Geometry check sheet. Reference: the model listing, model coordinates, mm. A direction names the side the tool comes from. Give positions to 0.01 mm unless a question says otherwise; leave off trailing zeros. Write each loop counter-clockwise with the first axis right and the second up, starting at its lowest first coordinate (ties: lowest second). Pieces come first, ordered by that corner, then holes.
(1) Thickness scan on line 1 along Z through (x, y) = (95.75, 19.6); line 2 along X through (y, z) = (15, 0); line 3 along X through (y, z) = (19.7, -13.75). Record the ranges inside material, lowest first.
(2) Cross-section at D-D (y = 12). Record the boundary of the cut face in (x, z).
(3) Cross-section at C-C (z = 0). Record the boundary of the cut face in (x, y), and give its area (4 significant figures).
(4) Mould release check, pull along Z, two halves, no side actions. Record for faces 5 (the flat face through (0, 4, 65.5)), 6 (the flat face through (2.5, 3, 68)), 7 (the flat face through (58, 16, 4.5)): +Z half, -Z half, draft (parallel to the pull), parting line (faces both ways), or undercut.
(5) Cross-section at A-A (x = 95.75). Record the boundary of the cut face in (y, z).
(6) Depth check by flat-ended pin: P1, Ø5, axis at y = 2.5, z = -67.5, coming from the +X side; P2, Ø1.5, axis at y = 3.5, z = 24, coming from the +X side; P3, Ø8, axis at x = -31, y = 6.5, coming from the -Z side; P4, Ø14, axis at x = 95.75, z = -13.75, coming from the -Y side. Enter the tip coordinate at first touch or a pass-through.
(7) Cross-section at B-B (x = 0). Record the boundary of the cut face in (y, z).
(8) Tool access check on faces 1 (the flat face through (-3, 20, 57)), 2 (the flat face through (0, 7, -68)), 3 (the flat face through (-2.5, 4, 68)), 4 (the flat face through (84, 19, 0)). Record the directions out of +Z, -Z, +X, -X, +Y, -Y that give a thin tool (end or side, any length) a straight path to the whole face; none if there is none.
Autodesk Inventor part; units mm, degrees
ref_plane "Pracovní rovina2" through (0, 0, 54.5) normal (0, 0, 1) x (1, 0, 0)
ref_plane "Pracovní rovina3" through (0, 0, -54.5) normal (0, 0, 1) x (1, 0, 0)
ref_plane "Pracovní rovina4" through (54.5, 0, 0) normal (1, 0, 0) x (0, 1, 0)
sketch "Náčrt1" plane through (0, 0, 0) normal (0, 1, 0) x (-1, 0, 0)
  circle A0 centre (0, 0) radius 55
  line L0 (0, -70) -> (26.9258, -70)
  line L1 (0, -70) -> (-26.9258, -70)
  line L2 (-70, 0) -> (-70, -26.9258)
  line L3 (-70, 0) -> (-70, 26.9258)
  line L4 (70, 0) -> (70, -26.9258)
  line L5 (70, 0) -> (70, 26.9258)
  line L6 (0, 70) -> (26.9258, 70)
  line L7 (0, 70) -> (-26.9258, 70)
  line L8 (-104.3981, 0) -> (104.3981, 0)
  line L9 (0, -104.3981) -> (0, 104.3981)
  arc A1 (26.9258, -70) -> (70, -26.9258) centre (0, 0) ccw
  arc A2 (-70, -26.9258) -> (-26.9258, -70) centre (0, 0) ccw
  arc A3 (70, 26.9258) -> (26.9258, 70) centre (0, 0) ccw
  arc A4 (-26.9258, 70) -> (-70, 26.9258) centre (0, 0) ccw
  dimension "d1" = 110
extrude "Vysunutí1" add sketch "Náčrt1" along normal blind 25 contours L8 L4 A1 L0 L9 A0 | A0 L9 L6 A3 L5 L8 | A0 L8 L3 A4 L7 L9 | L9 L1 A2 L2 L8 A0
sketch "Náčrt2" plane through (-26.9258, 0, 70) normal (0, 0, 1) x (1, 0, 0)
  line L0 (53.8516, 0) -> (0, 0)
  line L1 (24.4258, 0) -> (29.4258, 0)
  line L2 (29.4258, 0) -> (29.4258, 7)
  line L3 (29.4258, 7) -> (24.4258, 7)
  line L4 (24.4258, 7) -> (24.4258, 0)
  line L5 (96.9258, 0) -> (96.9258, 25)
  point P0 (26.9258, 0)
  dimension "d5" = 5
  dimension "d6" = 7
  dimension "d7" = 67.5
extrude "Vysunutí2" cut sketch "Náčrt2" against normal blind 4.5
sketch "Náčrt3" plane through (26.9258, 0, -70) normal (0, 0, -1) x (-1, 0, 0)
  line L0 (0, 0) -> (53.8516, 0)
  line L1 (53.8516, 0) -> (53.8516, 25)
  line L2 (0, 25) -> (53.8516, 25)
  line L3 (0, 0) -> (0, 25)
  line L4 (53.8516, 0) -> (96.9258, 0)
  line L5 (96.9258, 0) -> (96.9258, 25)
  line L6 (53.8516, 25) -> (96.9258, 25)
  line L7 (53.8516, 0) -> (53.8516, 25)
  line L8 (24.4258, 0) -> (0, 0)
  line L9 (24.4258, 0) -> (29.4258, 0)
  line L10 (29.4258, 0) -> (29.4258, 7)
  line L11 (29.4258, 7) -> (24.4258, 7)
  line L12 (24.4258, 7) -> (24.4258, 0)
  point P0 (26.9258, 0)
  dimension "d10" = 5
  dimension "d11" = 7
  dimension "d12" = 67.5
extrude "Vysunutí3" cut sketch "Náčrt3" against normal blind 4.5 contours L12 L11 L10 L0
sketch "Náčrt4" plane through (0, 25, 0) normal (0, 1, 0) x (1, 0, 0)
  line L0 (70, -26.9258) -> (70, 26.9258)
  line L1 (70, -4.5) -> (52.6737, -4.5)
  line L2 (52.6737, -4.5) -> (52.6737, 4.5)
  line L3 (52.6737, 4.5) -> (70, 4.5)
  line L4 (70, 4.5) -> (70, -4.5)
  line L5 (-98, 0) -> (98, 0)
  line L6 (0, 98) -> (0, -98)
  point P0 (0, 0)
  point P1 (70, 4.5)
  dimension "d15" = 9
  dimension "d16" = 4.5
extrude "Vysunutí4" cut sketch "Náčrt4" against normal blind 4
ref_plane "Pracovní rovina2" through (0, 0, 54.5) normal (0, 0, 1) x (1, 0, 0)
sketch "Náčrt6" plane through (0, 0, 54.5) normal (0, 0, 1) x (1, 0, 0)
  line L0 (-26.9258, 25) -> (26.9258, 25)
  line L1 (3, 25) -> (-3, 25)
  line L2 (-3, 25) -> (-3, 15)
  line L3 (-3, 15) -> (3, 15)
  line L4 (3, 15) -> (3, 25)
  line L5 (0, 30) -> (0, -5)
  point P0 (0, 0)
  dimension "d21" = 6
  dimension "d22" = 10
extrude "Vysunutí5" cut sketch "Náčrt6" along normal blind 4.5
ref_plane "Pracovní rovina3" through (0, 0, -54.5) normal (0, 0, 1) x (1, 0, 0)
sketch "Náčrt7" plane through (0, 0, -54.5) normal (0, 0, 1) x (1, 0, 0)
  line L0 (-55, 25) -> (54.8156, 25)
  line L1 (2.5, 25) -> (-2.5, 25)
  line L2 (-2.5, 25) -> (-2.5, 15)
  line L3 (-2.5, 15) -> (2.5, 15)
  line L4 (2.5, 15) -> (2.5, 25)
  line L5 (0, 30) -> (0, -5)
  point P0 (0, 0)
  point P1 (-3, 25)
  dimension "d26" = 5
  dimension "d27" = 10
extrude "Vysunutí6" cut sketch "Náčrt7" against normal blind 4.5
sketch "Náčrt8" plane through (70, 0, 26.9258) normal (1, 0, 0) x (0, 0, -1)
  line L0 (3.4258, 21) -> (50.4258, 21)
  line L1 (50.4258, 21) -> (50.4258, 19)
  line L2 (50.4258, 19) -> (3.4258, 19)
  line L3 (3.4258, 19) -> (3.4258, 21)
  line L4 (31.4258, 21) -> (22.4258, 21)
  line L5 (53.8516, 25) -> (0, 25)
  line L6 (26.9258, 25) -> (26.9258, 9.9917)
  point P0 (26.9258, 0)
  dimension "d30" = 47
  dimension "d31" = 2
extrude "Vysunutí7" add sketch "Náčrt8" along normal blind 37
sketch "Náčrt9" plane through (0, 21, 0) normal (0, 1, 0) x (1, 0, 0)
  circle A0 centre (95.75, -13.75) radius 8.75
  circle A1 centre (95.75, 13.75) radius 8.75
  line L0 (-105.4, 0) -> (142.4, 0)
  line L1 (107, 23.5) -> (107, -23.5)
  point P0 (0, 0)
  dimension "d34" = 17.5
  dimension "d35" = 17.5
  dimension "d37" = 5
  dimension "d38" = 5
  dimension "d41" = 11.25
  dimension "d42" = 11.25
extrude "Vysunutí8" cut sketch "Náčrt9" against normal blind 27
ref_plane "Pracovní rovina4" through (54.5, 0, 0) normal (1, 0, 0) x (0, 1, 0)
sketch "Náčrt10" plane through (54.5, 0, 0) normal (1, 0, 0) x (0, 1, 0)
  line L0 (0, 55) -> (0, -55)
  line L1 (21, -4.5) -> (0, -4.5)
  line L2 (0, -4.5) -> (0, 4.5)
  line L3 (0, 4.5) -> (21, 4.5)
  line L4 (21, 4.5) -> (21, -4.5)
  point P0 (0, 0)
  dimension "d44" = 9
extrude "Vysunutí9" cut sketch "Náčrt10" along normal blind 4
properties part number "Kruh"
Reply:
1. line 1: z = -23.5 to -22.5, -5 to 5, 22.5 to 23.5
1. line 2: x = -70 to -55, 58.5 to 70
1. line 3: x = -70 to -53.25, 53.25 to 87, 104.5 to 107
2. outline: (-70, -26.93) arc R75 ccw to (-26.93, -70) - (26.93, -70) arc R75 ccw to (70, -26.93) - (70, 26.93) arc R75 ccw to (26.93, 70) - (-26.93, 70) arc R75 ccw to (-70, 26.93) - close; hole (54.82, -4.5) - (58.5, -4.5) - (58.5, 4.5) - (54.82, 4.5) arc R55 ccw (long way) to start
3. outline: (-70, 0) - (-55, 0) - (-55, 25) - (-70, 25) - close; (58.5, 0) - (70, 0) - (70, 19) - (107, 19) - (107, 21) - (58.5, 21) - close
3. area: 690.5 mm2
4. face 5: +Z half
4. face 6: draft
4. face 7: undercut
5. outline: (19, -23.5) - (21, -23.5) - (21, -22.5) - (19, -22.5) - close; (19, -5) - (21, -5) - (21, 5) - (19, 5) - close; (19, 22.5) - (21, 22.5) - (21, 23.5) - (19, 23.5) - close
6. P1: stops at x = 37.42
6. P2: stops at x = 70
6. P3: stops at z = -69.97
6. P4: passes through
7. outline: (0, -65.5) - (7, -65.5) - (7, -70) - (25, -70) - (25, -59) - (15, -59) - (15, -55) - (0, -55) - close; (0, 55) - (15, 55) - (15, 59) - (25, 59) - (25, 70) - (7, 70) - (7, 65.5) - (0, 65.5) - close
8. face 1: +Y
8. face 2: -Z, -Y
8. face 3: +Z, -Y
8. face 4: +Z, -Z, +X, -Y
